Input: part model. Units: mm. Frame: model coordinates. Face numbers are marked on the shaded views. Give positions to 0.01 mm unless a question says otherwise; leave off trailing zeros. Loops run counter-clockwise (first coordinate to the right, second up) from the corner with the lowest first, then second, coordinate; pieces in that order, holes last. Notation, with made-up numbers: (-5.5, -0.5) - (18.5, -0.5) arc R22 cw to (18.5, 31.5) - close; hole circle Ø9 at (82.25, -16.75). An arc over 180 degrees is marked (long way). Answer as a JSON object with one key per item and string values.
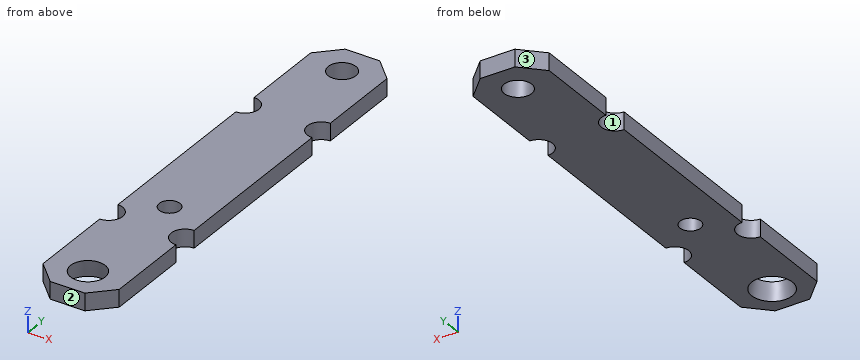
from build123d import *

# Parameters (mm, degrees)
ESQUISSE1_R      = 4
ESQUISSE1_R_2    = 3
EXTRUSION1_DEPTH = 5


with BuildPart() as part:
    # Esquisse1 → Extrusion1 (new body)
    with BuildSketch(Plane.XY):
        with BuildLine():
            Line((-5, 65), (5, 65))
            Line((5, 65), (11, 59))
            Line((11, 59), (11, 34))
            ThreePointArc((11, 34), (7, 30), (11, 26))
            Line((11, 26), (11, -26))
            ThreePointArc((11, -26), (7, -30), (11, -34))
            Line((11, -34), (11, -59))
            Line((11, -59), (5, -65))
            Line((5, -65), (-5, -65))
            Line((-5, -65), (-11, -59))
            Line((-11, -59), (-11, -34))
            ThreePointArc((-11, -34), (-7, -30), (-11, -26))
            Line((-11, -26), (-11, 26))
            ThreePointArc((-11, 26), (-7, 30), (-11, 34))
            Line((-11, 34), (-11, 59))
            Line((-11, 59), (-5, 65))
        make_face()
        with Locations((0, 56)):
            Circle(ESQUISSE1_R, mode=Mode.SUBTRACT)
        with Locations((0, -20)):
            Circle(ESQUISSE1_R_2, mode=Mode.SUBTRACT)
    extrude(amount=EXTRUSION1_DEPTH)

    # Esquisse2 → Enlèvement de matière-Révolution1 (revolve, cut)
    with BuildSketch(Plane(origin=(0, 0, 0), x_dir=(0, 0, -1), z_dir=(1, 0, 0)), mode=Mode.PRIVATE) as enl_vement_de_mati_re_r_volution1_sk:
        Polygon((-5, -51), (0, -50.118365096), (0, -52.065498843), (0, -56), (-5, -56), align=None)
    revolve(enl_vement_de_mati_re_r_volution1_sk.sketch.rotate(Axis((0, -56, -5.75818426), (0, 0, 1)), 90), axis=Axis((0, -56, -5.75818426), (0, 0, 1)), mode=Mode.SUBTRACT)


solid = part.part
Item 1: Cut plane A-A (y = -20). Return loops of the section in (x, z).
Geometry check:
{"outline": "(-11, 0) - (-3, 0) - (-3, 5) - (-11, 5) - close; (3, 0) - (11, 0) - (11, 5) - (3, 5) - close"}
Item 2: Cut plane D-D (z = 2). Return loops of the section in (x, y), then the cut area to 3 significant figures.
Geometry check:
{"outline": "(-11, -59) - (-5, -65) - (5, -65) - (11, -59) - (11, -34) arc R4 cw to (11, -26) - (11, 26) arc R4 cw to (11, 34) - (11, 59) - (5, 65) - (-5, 65) - (-11, 59) - (-11, 34) arc R4 cw to (-11, 26) - (-11, -26) arc R4 cw to (-11, -34) - close; hole circle Ø11.06 at (0, -56); hole circle Ø8 at (0, 56); hole circle Ø6 at (0, -20)", "area": "2,510 mm2"}
Item 3: Cut plane C-C (x = 9). Return loops of the section in (y, z), then the cut area to 3 significant figures.
Geometry check:
{"outline": "(-61, 0) - (-33.46, 0) - (-33.46, 5) - (-61, 5) - close; (-26.54, 0) - (26.54, 0) - (26.54, 5) - (-26.54, 5) - close; (33.46, 0) - (61, 0) - (61, 5) - (33.46, 5) - close", "area": "541 mm2"}
Item 4: Cut plane B-B (x = 0). Return loops of the section in (y, z), then the cut area to 3 significant figures.
Geometry check:
{"outline": "(-65, 0) - (-61.88, 0) - (-61, 5) - (-65, 5) - close; (-51, 5) - (-50.12, 0) - (-23, 0) - (-23, 5) - close; (-17, 0) - (52, 0) - (52, 5) - (-17, 5) - close; (60, 0) - (65, 0) - (65, 5) - (60, 5) - close", "area": "526 mm2"}
Item 5: Contact query for flat-ended pins moving along their axis: P1, Ø3.5, axis at x = 0, y = -20, coming from the +Z side; P2, Ø1.5, axis at x = -8.5, z = 3.5, coming from the -Y side; P3, Ø1, axis at x = 6.5, y = 50, coming from the -Z side. Output: stop coordinate, or through.
Geometry check:
{"P1": "passes through", "P2": "stops at y = -62.25", "P3": "stops at z = 0"}
Item 6: Mould query, pull axis Y, two halves, no side actions, for the marked faces 1, 2 and 3. Classes: released by +Y, released by -Y, zero draft, split by the parting line, or undercut.
Geometry check:
{"face 1": "undercut", "face 2": "released by -Y", "face 3": "released by +Y"}
Item 7: Material intervals for line 1 (Y direction, x = 0.5, z = 1.25); line 2 (Y direction, x = 9.25, z = 4.8); line 3 (Y direction, x = 3.5, z = 4.2), sorted ascending. Write a range as [from, to].
Geometry check:
{"line 1": "y = [-65, -61.64], [-50.36, -22.96], [-17.04, 52.03], [59.97, 65]", "line 2": "y = [-60.75, -33.6], [-26.4, 26.4], [33.6, 60.75]", "line 3": "y = [-65, -59.77], [-52.23, 54.06], [57.94, 65]"}
